Can you work these out from the model? Positions are in its coordinate system, mm. Face numbers are marked on the shaded views. A direction names the side the tool comes from. Give positions to 0.01 mm unless a question says otherwise; leave off trailing zeros. Order: outer loops, then holes, each group sorted by start corner. A loop starts at its lowest first (then second) coordinate and runs counter-clockwise, first axis right, second up. Notation, with made-up numbers: (39, 12) - (94, 12) arc R11 ccw to (94, 29) - close; hole circle Ø6 at (6.25, -5). An arc over 180 degrees is marked (long way). Write each question's results on one line, items separated by ' | '. Start each with the question number.
Autodesk Inventor part; units mm, degrees
ref_plane "YZ Plane" through (0, 0, 0) normal (1, 0, 0) x (0, 1, 0)
ref_plane "XZ Plane" through (0, 0, 0) normal (0, 1, 0) x (-1, 0, 0)
ref_plane "XY Plane" through (0, 0, 0) normal (0, 0, 1) x (1, 0, 0)
sketch "Esquisse1" plane through (0, 0, 0) normal (0, 0, 1) x (1, 0, 0)
  point P0 (0, 0)
sketch "Esquisse2" plane through (0, 0, 0) normal (0, 0, 1) x (1, 0, 0)
  circle A0 centre (0, 0) radius 17.5
  circle A1 centre (0, 0) radius 14
  dimension "d0" = 35
  dimension "d1" = 28
extrude "Extrusion1" add sketch "Esquisse2" along normal blind 74
sketch "Esquisse3" plane through (0, 0, 0) normal (0, 0, -1) x (-1, 0, 0)
  line L0 (2.4577, 17.3266) -> (2.4577, 67.3266)
  line L1 (2.4577, 67.3266) -> (-2.4577, 67.3266)
  line L2 (-2.4577, 67.3266) -> (-2.4577, 17.3266)
  circle A0 centre (0, 0) radius 17.5
  arc A1 (2.4577, 17.3266) -> (-2.4577, 17.3266) centre (0, 0) ccw
  dimension "d4" = 50
extrude "Extrusion2" add sketch "Esquisse3" against normal blind 100 contours A0 L2 L1 L0
sketch "Esquisse4" plane through (2.4577, 17.3266, 0) normal (1, 0, 0) x (0, 0, -1)
  point P0 (0, -17.3266)
sketch "Esquisse5" plane through (2.4577, 17.3266, 0) normal (1, 0, 0) x (0, 0, -1)
  point P0 (0, -17.3266)
sketch "Esquisse6" plane through (2.4577, 17.3266, 0) normal (1, 0, 0) x (0, 0, -1)
  line L0 (-74, 0) -> (-74, -34.8266)
  line L1 (-100, 0) -> (-100, 50)
  arc A0 (-74, 0) -> (-100, 38.4236) centre (-128.4832, -8.8585) ccw
  line L2 (-100, 38.4236) -> (-100, 0)
  line L3 (-74, 0) -> (-100, 0)
  line L4 (-74, 0) -> (-100, 0)
  point P0 (0, -17.3266)
extrude "Extrusion3" cut sketch "Esquisse6" against normal blind 31
sketch "Esquisse7" plane through (2.4577, 17.3266, 0) normal (1, 0, 0) x (0, 0, -1)
  line L0 (0, 0) -> (0, 50)
  line L1 (0, 50) -> (-100, 50)
  arc A0 (0, 0) -> (-70.9999, 50) centre (-205.1565, -215.912) ccw
  point P0 (0, -17.3266)
extrude "Extrusion4" cut sketch "Esquisse7" against normal blind 19.75
pattern_circular "Réseau circulaire1" count 3 over 360 about axis through (0, 0, 0) along (0, 0, 1) of "Extrusion2", "Extrusion4", "Extrusion3"
fillet "Congé1" radius 2 6 edges at (-16.2341, -6.5349, 37) (-2.4577, 17.3266, 37) (2.4577, 17.3266, 37) (16.2341, -6.5349, 37) (13.7764, -10.7917, 37) (-13.7764, -10.7917, 37)
properties part number "RocketBaseThing"
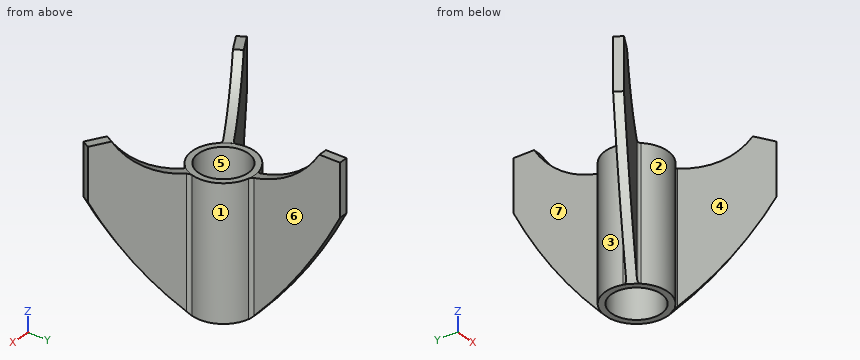
Q1. Will these pins go through, and if not, where does the flat tip stop? P1, Ø10, axis at y = -20, z = 17.5, coming from the +X side; P2, Ø24, axis at y = 47, z = 55.5, coming from the -X side; P3, Ø3, axis at x = -10.5, z = 49.5, coming from the +Y side.
Q2. Which directions (+Z, -Z, +X, -X, +Y, -Y) give clear straight access to the entire face, cutting with the end or side of a thin tool? Please do the marked faces 4, 5, 6 and 7.
Q3. If I drill on probe 1 along X at (y, z) = (26.5, 13); probe 2 along X at (y, z) = (-28.5, 61.5); probe 3 along Y at (x, z) = (0, 42), over which ranges is the centre line in solid material (lowest first)? Write a range as from..to.
Q4. Thinking about a two-plate mould opening in X: for the marked faces 1, 2 and 3, which applies, released by +X, released by -X, zero draft, split by the parting line, or undercut?
Q5. If we section it at A-A (y = 0): Please give me the cut outline in (x, z), plus the area to 3 significant figures.
Q6. If we section it at D-D (z = 80.5): Please give me the cut outline in (x, y).
Q7. If we section it at C-C (z = 44): Please give me the cut outline in (x, y), plus the area to 3 significant figures.
Findings below:
1) P1: stops at x = 31.64 | P2: stops at x = -2.46 | P3: stops at y = 15.01
2) face 4: +Z, -Z, -Y | face 5: +Z, -Z | face 6: +Z, -Z, +X, +Y | face 7: +Z, -Z, -X, +Y
3) probe 1: x = -2.46..2.46 | probe 2: x = -54.28..-44.45, 44.45..54.28 | probe 3: y = -17.5..-14, 14..50.59
4) face 1: released by +X | face 2: undercut | face 3: released by -X
5) outline: (-17.5, 0) - (-14, 0) - (-14, 74) - (-17.5, 74) - close; (14, 0) - (17.5, 0) - (17.5, 74) - (14, 74) - close | area: 518 mm2
6) outline: (-59.54, -31.53) - (-57.08, -35.79) - (-29.73, -20.01) - (-32.19, -15.75) - close; (-2.46, 35.75) - (2.46, 35.75) - (2.46, 67.33) - (-2.46, 67.33) - close; (29.73, -20.01) - (57.08, -35.79) - (59.54, -31.53) - (32.19, -15.75) - close
7) outline: (-46.16, -23.81) - (-43.71, -28.07) - (-15.21, -11.62) arc R2 cw to (-12.75, -11.98) arc R17.5 ccw to (12.75, -11.98) arc R2 cw to (15.21, -11.62) - (43.71, -28.07) - (46.16, -23.81) - (17.67, -7.36) arc R2 cw to (16.75, -5.05) arc R17.5 ccw to (4, 17.04) arc R2 cw to (2.46, 18.98) - (2.46, 51.89) - (-2.46, 51.89) - (-2.46, 18.98) arc R2 cw to (-4, 17.04) arc R17.5 ccw to (-16.75, -5.05) arc R2 cw to (-17.67, -7.36) - close; hole circle Ø28 at (0, 0) | area: 857 mm2
